Part model, mm, in its own coordinate system. A direction names the side the tool comes from. Round coordinates to 2 decimals unless told otherwise and drop trailing zeros. Write each loop counter-clockwise with the first axis right and the second up, starting at its lowest first coordinate (ties: lowest second). Pieces come first, ordered by that corner, then holes.
Autodesk Inventor part; units mm, degrees
ref_plane "YZ Plane" through (0, 0, 0) normal (1, 0, 0) x (0, 1, 0)
ref_plane "XZ Plane" through (0, 0, 0) normal (0, 1, 0) x (-1, 0, 0)
ref_plane "XY Plane" through (0, 0, 0) normal (0, 0, 1) x (1, 0, 0)
sketch "Sketch1" plane through (0, 0, 0) normal (0, 0, 1) x (1, 0, 0)
  line L0 (-15.7, 12.7) -> (-12.7, 12.7)
  line L1 (-12.7, 12.7) -> (-12.7, -9.7)
  line L2 (-12.7, -9.7) -> (12.7, -9.7)
  line L3 (12.7, -9.7) -> (12.7, 12.7)
  line L4 (12.7, 12.7) -> (15.7, 12.7)
  line L5 (15.7, 12.7) -> (15.7, -12.7)
  line L6 (15.7, -12.7) -> (-15.7, -12.7)
  line L7 (-15.7, -12.7) -> (-15.7, 12.7)
  point P0 (0, 0)
  dimension "d0" = 3
  dimension "d2" = 3
  dimension "d3" = 25.4
  dimension "d4" = 31.4
  dimension "d5" = 15.7
  dimension "d7" = 12.7
  dimension "d8" = 3
extrude "Extrusion1" add sketch "Sketch1" against normal blind 381
equation "\"d2\" = d0"
equation "\"d8\" = d0"
properties part number "15in c channel"
Q1. Cut at A-A on y = -5.5. Write the cut outline in (x, z).
Values follow:
outline: (-15.7, -381) - (-12.7, -381) - (-12.7, 0) - (-15.7, 0) - close; (12.7, -381) - (15.7, -381) - (15.7, 0) - (12.7, 0) - close
Q2. Cut at B-B on z = -168.5. Write the cut outline in (x, y).
Values follow:
outline: (-15.7, -12.7) - (15.7, -12.7) - (15.7, 12.7) - (12.7, 12.7) - (12.7, -9.7) - (-12.7, -9.7) - (-12.7, 12.7) - (-15.7, 12.7) - close
Q3. Drop a flat-ended pin along its axis: pin 1 (4 mm diameter, centred on x = 3, z = -239, fed in from +Y). Give the stop position or say it passes through.
Values follow:
pin 1: stops at y = -9.7
Q4. Mould opens along X. For faces 3 (the flat face through (-15.7, 0, -188)), 4 (the flat face through (-12.7, 2, -188)), 5 (the flat face through (0, -12.7, -188)) say: +X half, -X half, draft (parallel to the pull), parting line (faces both ways), or undercut.
Values follow:
face 3: -X half
face 4: undercut
face 5: draft
Q5. Wall check: L1, parallel to X at y = 6, z = -293; L2, parallel to Y at x = -8, z = -255.5. Give the ranges that are in metal, low to high.
Values follow:
L1: x = -15.7 to -12.7, 12.7 to 15.7
L2: y = -12.7 to -9.7
Q6. Cut at C-C on x = 7.5. Write the cut outline in (y, z), plus the area to 3 significant figures.
Values follow:
outline: (-12.7, -381) - (-9.7, -381) - (-9.7, 0) - (-12.7, 0) - close
area: 1,140 mm2
Q7. Which spindle directions (+Z, -Z, +X, -X, +Y, -Y) get a long thin tool onto all of the face, cutting with end or side? Do faces 1 (the flat face through (12.7, 1, -188)), 2 (the flat face through (0, -10, 0)). Say none if no direction does.
Values follow:
face 1: +Z, -Z, +Y
face 2: +Z, +X, -X, +Y, -Y
